For this review, take the finished solid that the model builds, in its own axes (mm). Coordinates: 2 decimals unless noted, no trailing zeros. Loops run counter-clockwise (first coordinate to the right, second up) from the corner with the lowest first, then second, coordinate; pieces in that order, holes last.
1. To check wall thickness, follow probe 1 along Y at (x, z) = (-15.5, 0.4); probe 2 along Y at (x, z) = (-1.5, 0.25); probe 3 along X at (y, z) = (40, 1.05). State the ranges of each line that lie inside material, in increasing order.
2. Take a section at D-D, the plane z = 0.8. Count the separate pieces of the cut face and the enclosed holes in it, then the cut area to 3 significant figures.
3. Take a section at C-C, the plane y = -31. State the section outline as (x, z) points.
4. Take a section at A-A, the plane y = 40. State the section outline as (x, z) points.
5. Take a section at B-B, the plane x = 2.5. State the section outline as (y, z) points, then the cut area to 3 significant figures.
```python
from build123d import *

# Parameters (mm, degrees)
SKETCH1_W           = 44
SKETCH1_H           = 100
BOSS_EXTRUDE1_DEPTH = 2
SKETCH2_R           = 1.5
CUT_EXTRUDE1_DEPTH  = 2
SKETCH3_W           = 18
SKETCH3_H           = 5
CUT_EXTRUDE2_DEPTH  = 10
SKETCH4_R           = 1.5
SKETCH4_W           = 12
SKETCH4_H           = 5
SKETCH4_W_2         = 8
CUT_EXTRUDE3_DEPTH  = 55.662601475


with BuildPart() as part:
    # Sketch1 → Boss-Extrude1 (new body)
    with BuildSketch(Plane.XY):
        Rectangle(SKETCH1_W, SKETCH1_H)
    extrude(amount=BOSS_EXTRUDE1_DEPTH)

    # Sketch2 → Cut-Extrude1 (cut)
    with BuildSketch(Plane.XY.offset(2)):
        with Locations((-8, -40)):
            Circle(SKETCH2_R)
        with Locations((18.5, -40)):
            Circle(SKETCH2_R)
        with Locations(Location((18.5, -13.5, 0), (0, 0, 180))):
            Circle(SKETCH2_R)
        with Locations(Location((-8, -13.5, 0), (0, 0, 180))):
            Circle(SKETCH2_R)
        with Locations(Location((18.5, 40, 0), (0, 0, 180))):
            Circle(SKETCH2_R)
        with Locations(Location((-8, 40, 0), (0, 0, 180))):
            Circle(SKETCH2_R)
        with Locations((18.5, 13.5)):
            Circle(SKETCH2_R)
        with Locations((-8, 13.5)):
            Circle(SKETCH2_R)
    extrude(amount=-CUT_EXTRUDE1_DEPTH, mode=Mode.SUBTRACT)

    # Sketch3 → Cut-Extrude2 (cut)
    with BuildSketch(Plane.XY.offset(2)):
        with Locations((5, 40.5)):
            Rectangle(SKETCH3_W, SKETCH3_H)
        with Locations((5, 13.004717401)):
            Rectangle(SKETCH3_W, SKETCH3_H)
        with Locations((5, -13.004717401)):
            Rectangle(SKETCH3_W, SKETCH3_H)
        with Locations((5, -40.5)):
            Rectangle(SKETCH3_W, SKETCH3_H)
    extrude(amount=-CUT_EXTRUDE2_DEPTH, mode=Mode.SUBTRACT)

    # Sketch4 → Cut-Extrude3 (cut, through all)
    with BuildSketch(Plane.XY.offset(2)):
        with Locations((-18.5, -31)):
            Circle(SKETCH4_R)
        with Locations((-14, -22.5)):
            Rectangle(SKETCH4_W, SKETCH4_H)
        with Locations((-12, -30.746090286)):
            Rectangle(SKETCH4_W_2, SKETCH4_H)
    extrude(amount=-CUT_EXTRUDE3_DEPTH, mode=Mode.SUBTRACT)


solid = part.part
```
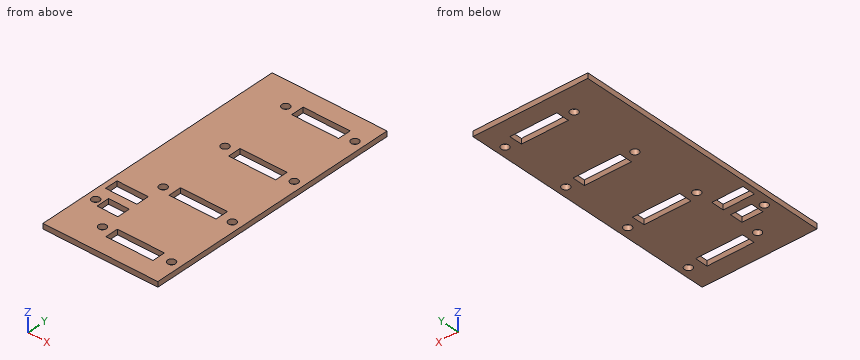
Results list:
1. probe 1: y = -50 to -33.25, -28.25 to -25, -20 to 50
1. probe 2: y = -50 to -43, -38 to -15.5, -10.5 to 10.5, 15.5 to 38, 43 to 50
1. probe 3: x = -22 to -9.5, -6.5 to -4, 14 to 17, 20 to 22
2. separate pieces: 1
2. enclosed holes: 15
2. area: 3,880 mm2
3. outline: (-22, 0) - (-20, 0) - (-20, 2) - (-22, 2) - close; (-17, 0) - (-16, 0) - (-16, 2) - (-17, 2) - close; (-8, 0) - (22, 0) - (22, 2) - (-8, 2) - close
4. outline: (-22, 0) - (-9.5, 0) - (-9.5, 2) - (-22, 2) - close; (-6.5, 0) - (-4, 0) - (-4, 2) - (-6.5, 2) - close; (14, 0) - (17, 0) - (17, 2) - (14, 2) - close; (20, 0) - (22, 0) - (22, 2) - (20, 2) - close
5. outline: (-50, 0) - (-43, 0) - (-43, 2) - (-50, 2) - close; (-38, 0) - (-15.5, 0) - (-15.5, 2) - (-38, 2) - close; (-10.5, 0) - (10.5, 0) - (10.5, 2) - (-10.5, 2) - close; (15.5, 0) - (38, 0) - (38, 2) - (15.5, 2) - close; (43, 0) - (50, 0) - (50, 2) - (43, 2) - close
5. area: 160 mm2
